The listing builds one solid part. Answer for the finished solid, in the listing's coordinates (mm). Face numbers are marked on the shaded views. A direction names the side the tool comes from. Give positions to 0.01 mm unless a question says otherwise; leave off trailing zeros. Loops run counter-clockwise (first coordinate to the right, second up) from the corner with the lowest first, then second, coordinate; pieces in that order, holes last. Notation, with made-up numbers: M 78,54.25 L 126,54.25 A13 cw 126,79.25 Z; hole C 6,59.5 d1. An arc over 180 degrees is marked long. Return JSON: item names as keys, results as strings.
from build123d import *

# Parameters (mm, degrees)
EXTRUDE_THIN1_DEPTH = 53.975
BOSS_EXTRUDE1_START = 27.94
BOSS_EXTRUDE1_DEPTH = 19.05
BOSS_EXTRUDE2_DEPTH = 28.194
SKETCH12_W          = 34.867415814
SKETCH12_H          = 30.773507234
CUT_EXTRUDE1_DEPTH  = 27.000736901
SKETCH13_W          = 2.54
SKETCH13_H          = 35.56
BOSS_EXTRUDE3_DEPTH = 16.51
SKETCH14_W          = 72.898
SKETCH14_H          = 6.223180908
BOSS_EXTRUDE4_DEPTH = 2.54


with BuildPart() as part:
    # Sketch8 → Extrude-Thin1 (new body)
    with BuildSketch(Plane(origin=(0, 0, 0), x_dir=(1, 0, 0), z_dir=(0, 1, 0))):
        with BuildLine():
            ThreePointArc((-21.840673053, -0.381230366), (-15.310661969, -15.580242811), (0, -21.844))
            Line((0, -21.844), (72.898, -21.844))
            ThreePointArc((72.898, -21.844), (85.209931142, -16.744231142), (90.3097, -4.4323))
            Line((90.3097, -4.4323), (92.8497, -4.4323))
            ThreePointArc((92.8497, -4.4323), (87.005982366, -18.540282366), (72.898, -24.384))
            Line((72.898, -24.384), (0, -24.384))
            ThreePointArc((0, -24.384), (-17.090971501, -17.391898952), (-24.380286199, -0.425559479))
            Line((-24.380286199, -0.425559479), (-21.840673053, -0.381230366))
        make_face()
    extrude(amount=EXTRUDE_THIN1_DEPTH)

    # Sketch10 → Boss-Extrude1 (add)
    with BuildSketch(Plane(origin=(0, 0, 0), x_dir=(1, 0, 0), z_dir=(0, 1, 0)).offset(BOSS_EXTRUDE1_START)):
        with BuildLine():
            Line((-6.641231784, -11.936352934), (-4.843541474, -10.138662625))
            Line((-4.843541474, -10.138662625), (-3.045851165, -11.936352934))
            Line((-3.045851165, -11.936352934), (-5.383859486, -15.696211745))
            ThreePointArc((-5.383859486, -15.696211745), (-7.807213542, -17.931410627), (-10.959862847, -18.895548216))
            ThreePointArc((-10.959862847, -18.895548216), (-15.446040528, -15.446040528), (-18.895548216, -10.959862847))
            ThreePointArc((-18.895548216, -10.959862847), (-17.931410627, -7.807213542), (-15.696211745, -5.383859486))
            Line((-15.696211745, -5.383859486), (-11.936352934, -3.045851165))
            Line((-11.936352934, -3.045851165), (-10.138662625, -4.843541474))
            Line((-10.138662625, -4.843541474), (-11.936352934, -6.641231784))
            ThreePointArc((-11.936352934, -6.641231784), (-14.946738288, -14.946738288), (-6.641231784, -11.936352934))
        make_face()
    extrude(amount=BOSS_EXTRUDE1_DEPTH)

    # Sketch11 → Boss-Extrude2 (add)
    with BuildSketch(Plane(origin=(0, 0, 0), x_dir=(1, 0, 0), z_dir=(0, 1, 0))):
        with BuildLine():
            Line((90.3097, -4.4323), (92.8497, -4.4323))
            Line((92.8497, -4.4323), (92.8497, 74.676))
            ThreePointArc((92.8497, 74.676), (91.491251092, 81.505383841), (87.622715901, 87.295055901))
            Line((87.622715901, 87.295055901), (85.826664677, 85.499004677))
            ThreePointArc((85.826664677, 85.499004677), (89.14459708, 80.533367923), (90.3097, 74.676))
            Line((90.3097, 74.676), (90.3097, -4.4323))
        make_face()
    extrude(amount=BOSS_EXTRUDE2_DEPTH)

    # Sketch12 → Cut-Extrude1 (cut, through all)
    with BuildSketch(Plane(origin=(0, 0, 0), x_dir=(-0.999847695, 0, 0.017452406), z_dir=(-0.017452406, 0, -0.999847695))):
        with Locations((17.814938273, 11.918246383)):
            Rectangle(SKETCH12_W, SKETCH12_H)
    extrude(amount=-CUT_EXTRUDE1_DEPTH, mode=Mode.SUBTRACT)

    # Sketch13 → Boss-Extrude3 (add)
    with BuildSketch(Plane(origin=(0, 28.194, 0), x_dir=(1, 0, 0), z_dir=(0, 1, 0))):
        with Locations((91.5797, 13.3477)):
            Rectangle(SKETCH13_W, SKETCH13_H)
    extrude(amount=BOSS_EXTRUDE3_DEPTH)

    # Sketch14 → Boss-Extrude4 (add)
    with BuildSketch(Plane(origin=(0, 53.975, 0), x_dir=(1, 0, 0), z_dir=(0, 1, 0))):
        with Locations((36.449, -21.272409546)):
            Rectangle(SKETCH14_W, SKETCH14_H)
    extrude(amount=BOSS_EXTRUDE4_DEPTH)


solid = part.part
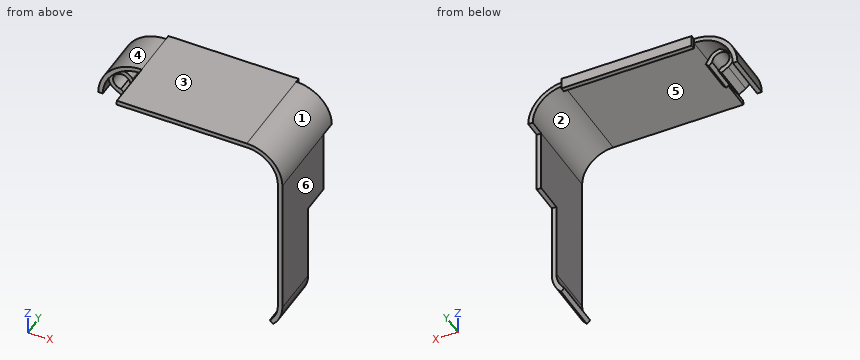
(1) A tool of negligible diameter and unlimited length cuts with its end or side. For the marked faces 5 and 6, from which of +Z, -Z, +X, -X, +Y, -Y can it reach the whole face along a straight path? Write none if from no direction.
Values follow:
{"face 5": "-Z, -Y", "face 6": "+Z, -Z, +X, +Y, -Y"}
(2) Given pin 1 (8 mm diameter, centred on x = 48.5, y = 29, fed in from -Z); pin 2 (1.3 mm diameter, centred on x = 34, y = 55.5, fed in from -Z); pin 3 (17.5 mm diameter, centred on x = -14.5, z = 11.5, fed in from +Y) (3 decimals); pin 4 (9 mm diameter, centred on x = -11.5, z = 11.5, fed in from +Y), each flat-ended and moving along its own axis, determine where each tip first touches the part or whether it passes through.
Values follow:
{"pin 1": "z = 21.84", "pin 2": "z = 18.16", "pin 3": "y = 53.975", "pin 4": "through"}
(3) Straight lines are drawn through the part: line 1 along Z through (x, y) = (9.5, 4); line 2 along Y through (x, z) = (-8, 17.5); line 3 along X through (y, z) = (20, -4). For each, find the intervals that lie inside material, in ascending order.
Values follow:
{"line 1": "21.84 to 24.38", "line 2": "27.94 to 46.99", "line 3": "90.31 to 92.85"}
(4) The part is cut by section C-C (z = -24.5). Determine the outline of the cut face in (x, y).
Values follow:
{"outline": "M 90.31,0 L 92.85,0 L 92.85,44.7 L 90.31,44.7 Z"}
(5) Determine the mould class of the marked faces 1, 2, 3 and 4 for opening direction X: released by +X, released by -X, zero draft, split by the parting line, or undercut.
Values follow:
{"face 1": "released by +X", "face 2": "undercut", "face 3": "zero draft", "face 4": "released by -X"}
(6) The part is cut by section D-D (y = 42). Determine the outline of the cut face in (x, z).
Values follow:
{"outline": "M -24.38,0.43 L -21.84,0.38 A21.84 cw -18.9,10.96 A7.42 ccw -15.7,5.38 L -11.94,3.05 L -10.14,4.84 L -11.94,6.64 A4.88 cw long -6.64,11.94 L -4.84,10.14 L -3.05,11.94 L -5.38,15.7 A7.42 ccw -10.96,18.9 A21.84 cw 0,21.84 L 72.9,21.84 A17.41 cw 90.31,4.43 L 90.31,-31.13 L 92.85,-31.13 L 92.85,4.43 A19.95 ccw 72.9,24.38 L 0,24.38 A24.38 ccw Z"}
(7) The part is cut by section A-A (y = 49). Determine the outline of the cut face in (x, z), and give its area (3 significant figures).
Values follow:
{"outline": "M -24.38,0.43 L -21.84,0.38 A21.84 cw 0,21.84 L 72.9,21.84 A17.41 cw 90.31,4.43 L 92.85,4.43 A19.95 ccw 72.9,24.38 L 0,24.38 A24.38 ccw Z", "area": "351 mm²"}
(8) The part is cut by section B-B (x = 42). Determine the outline of the cut face in (y, z) (3 decimals), and give its area (3 significant figures).
Values follow:
{"outline": "M 0,21.844 L 53.975,21.844 L 53.975,18.161 L 56.515,18.161 L 56.515,24.384 L 0,24.384 Z", "area": "153 mm²"}
